Verification items for this drawing (mm, ordinates from the low corner). Coordinates: 2 decimals unless noted, no trailing zeros. Order: outer loops, then holes, each group sorted by start corner. A loop starts at its lowest first (then second) coordinate and runs counter-clockwise, first axis right, second up. Notation, with made-up numbers: (20, -15) -> (42, -15) arc R11 ccw to (42, -7) -> close; hole circle Ø11 at (-10.5, 68.5). An arc over 180 degrees is marked (long way). Write each question's results on one line, items separated by ' | '. Start each with the question number.
(1) Cross-section at C-C on z = 0.75. Enter the section's corners in (x, y), and give its area (3 significant figures).
(2) Cross-section at B-B on z = 4.5. Enter the section's corners in (x, y) (1 decimal), and give its area (3 significant figures).
(3) Draft check along X on the marked faces 1, 2, 3 and 4. Enter one of: +X half, -X half, draft (parallel to the pull), parting line (faces both ways), or undercut.
(4) Go/stop test with flat-tipped pins: pin 1 (2 mm diameter, centred on x = 4.5, y = 5.5, fed in from -Z); pin 2 (1.5 mm diameter, centred on x = 1, z = 2.5, fed in from +Y). Record where each tip stops, or that it passes through.
(5) Cross-section at A-A on x = 6.5. Give the number of separate pieces and of enclosed holes in the cut face.
(6) Thickness scan on probe 1 along X at (y, z) = (5.5, 3.5) (1 decimal); probe 2 along X at (y, z) = (4, 1.5) (1 decimal); probe 3 along Y at (x, z) = (4.5, 1.25). Record the ranges inside material, lowest first. Write a range as [from, to].
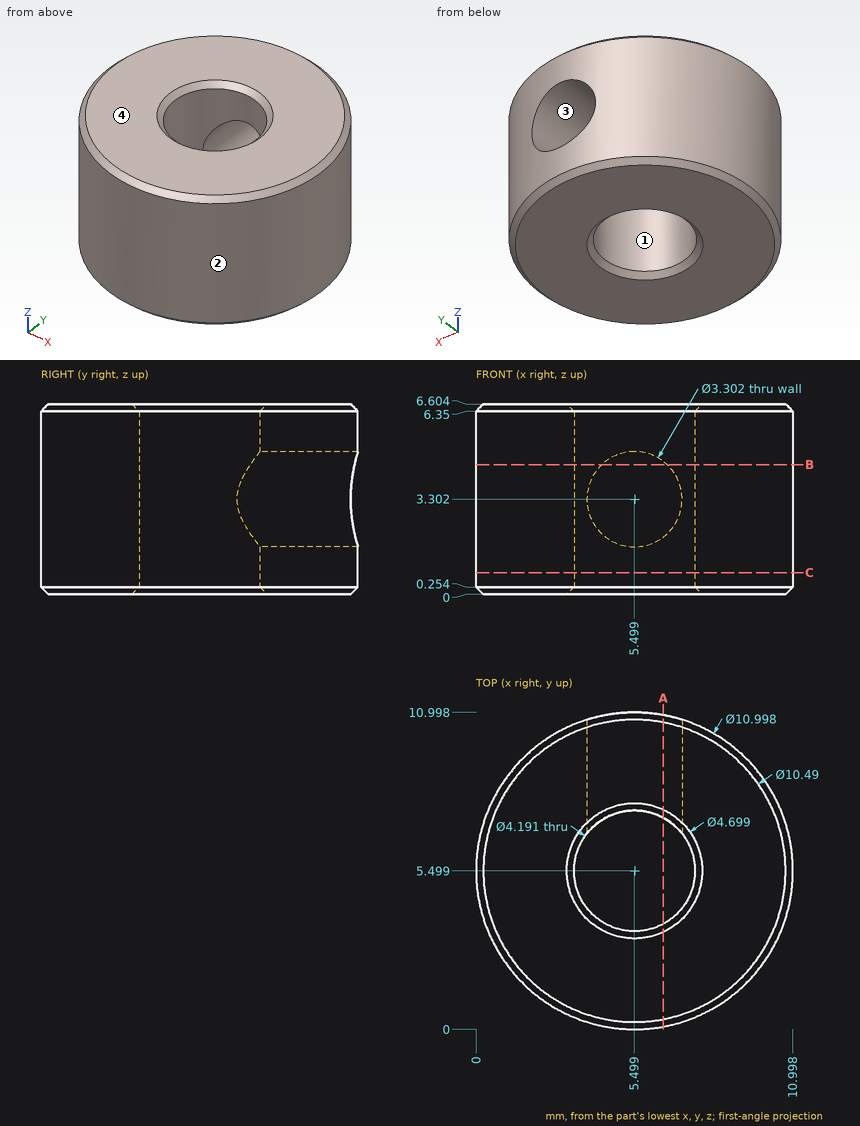
Results are:
1) outline: circle Ø11 at (5.5, 5.5); hole circle Ø4.19 at (5.5, 5.5) | area: 81.2 mm2
2) outline: (4.4, 7.3) -> (4.4, 10.9) arc R5.5 ccw (long way) to (6.6, 10.9) -> (6.6, 7.3) arc R2.1 cw (long way) to start | area: 73.3 mm2
3) face 1: undercut | face 2: parting line | face 3: undercut | face 4: draft
4) pin 1: passes through | pin 2: stops at y = 9.52
5) separate pieces: 3 | enclosed holes: 0
6) probe 1: x = [0, 3.4], [7.6, 11] | probe 2: x = [0.2, 4], [7, 10.8] | probe 3: y = [0.09, 3.66], [7.34, 10.91]
